Check sheet for the modelled part. Datum: model origin and axes. Units: mm. A direction names the side the tool comes from. Give positions to 0.01 mm unless a question says otherwise; leave off trailing zeros. Write each loop counter-clockwise with the first axis right and the second up, starting at its lowest first coordinate (ties: lowest second). Pieces come first, ordered by that corner, then holes. Notation, with made-up numbers: M 8.5,14 L 28.5,14 A25 ccw 28.5,35 Z; hole C 35,-21 d7. An arc over 180 degrees is marked long. Write item = value, one per line. Start each with the question number.
1) Scan lines: L1, parallel to Z at x = 293, y = 302; L2, parallel to Y at x = 222, z = 1.5; L3, parallel to X at y = 108.5, z = 1. Record each from-to range of solid material in increasing order.
2) Sectioned sample at A-A, the plane y = 333. Record the cut outline in (x, z), then the cut area to 3 significant figures.
3) Sectioned sample at B-B, the plane z = -5. Record the cut outline in (x, y), then the cut area to 3 significant figures.
4) Draft check along Y on faces 1 (the face through (281.901, 335.277, 1.479)), 2 (the face through (267.89, 313.772, 1.479)), 3 (the face through (189.3, 351.9, 1.5)), 4 (the face through (398.584, 56.784, 1.479)). Enter one of: pulls with the +Y half, pulls with the -Y half, needs draft (parallel to the pull), parting line crosses it, or undercut.
5) Set-up check for faces 5 (the face through (208.47, 362.55, 1.48)), 6 (the face through (346.985, 311.588, 1.479)), 7 (the face through (398.838, 182.595, -14.133)): record each of +Z, -Z, +X, -X, +Y, -Y from which the full face is reachable in a straight line by a thin tool's end or side.
6) Gauge pin test, flat ends, axial feed: pin 1 (5 mm diameter, centred on y = 116, z = -8.5, fed in from +X); pin 2 (3 mm diameter, centred on y = 113, z = -23, fed in from -X); pin 3 (6 mm diameter, centred on y = 322, z = -5.5, fed in from -X); pin 4 (4 mm diameter, centred on x = 312, y = 281, fed in from -Z). Record the tip position at first contact, or that the pin passes through.
from build123d import *

# Parameters (mm, degrees)
RESSALTO_EXTRUS_O1_DEPTH        = 3
ARESTA_FLANGE1_STRIP_W          = 13.8
ARESTA_FLANGE1_STRIP_H          = 3
ARESTA_FLANGE1_STRIP_CUT_DEPTH  = 248.223813341
ARESTA_FLANGE1_RELIEF_W         = 15.3
ARESTA_FLANGE1_RELIEF_H         = 1.5
ARESTA_FLANGE1_RELIEF_CUT_DEPTH = 3
ARESTA_FLANGE1_DEPTH            = 248.223813341


# Sheet-metal steps are written as plain solids
with BuildPart() as part:
    # Esboço29 → Ressalto-extrusão1 (new body)
    with BuildSketch(Plane.XY):
        with BuildLine():
            Line((423.645620755, 59.178719541), (380.542007914, 303.631455401))
            ThreePointArc((380.542007914, 303.631455401), (376.166741716, 313.014244041), (367.686255721, 318.952344263))
            Line((367.686255721, 318.952344263), (235.026475013, 367.236555725))
            ThreePointArc((235.026475013, 367.236555725), (228.186072146, 368.44270331), (221.34566928, 367.236555725))
            Line((221.34566928, 367.236555725), (195.221638123, 357.728185985))
            ThreePointArc((195.221638123, 357.728185985), (189.244913348, 351.75146121), (189.981585518, 343.331259777))
            Line((189.981585518, 343.331259777), (268.150737271, 207.938317356))
            ThreePointArc((268.150737271, 207.938317356), (270.383115212, 205.277872925), (273.390789876, 203.541391148))
            Line((273.390789876, 203.541391148), (294.669915314, 195.796422877))
            ThreePointArc((294.669915314, 195.796422877), (297.677589977, 194.059941101), (299.909967918, 191.399496669))
            Line((299.909967918, 191.399496669), (372.923716413, 64.935974625))
            ThreePointArc((372.923716413, 64.935974625), (375.848206088, 61.744454182), (379.847488675, 60.087897095))
            Line((379.847488675, 60.087897095), (417.853341101, 53.386439887))
            ThreePointArc((417.853341101, 53.386439887), (422.257115895, 54.774944746), (423.645620755, 59.178719541))
        make_face()
        with BuildLine():
            Line((243.325022214, 329.098265065), (239.916324262, 348.429951789))
            ThreePointArc((239.916324262, 348.429951789), (239.041271023, 350.306509517), (237.345173823, 351.494129561))
            Line((237.345173823, 351.494129561), (232.47795712, 353.265651565))
            ThreePointArc((232.47795712, 353.265651565), (231.109876546, 353.506881082), (229.741795973, 353.265651565))
            Line((229.741795973, 353.265651565), (204.889458572, 344.220140499))
            ThreePointArc((204.889458572, 344.220140499), (202.257539145, 340.461370016), (204.889458572, 336.702599533))
            Line((204.889458572, 336.702599533), (238.017710629, 324.644901871))
            ThreePointArc((238.017710629, 324.644901871), (241.956941641, 325.339494581), (243.325022214, 329.098265065))
        make_face(mode=Mode.SUBTRACT)
        with BuildLine():
            Line((249.39887944, 340.721872869), (252.807577392, 321.390186145))
            ThreePointArc((252.807577392, 321.390186145), (253.682630632, 319.513628417), (255.378727831, 318.326008373))
            Line((255.378727831, 318.326008373), (280.757120558, 309.089028826))
            ThreePointArc((280.757120558, 309.089028826), (282.125201132, 308.847799309), (283.493281705, 309.089028826))
            Line((283.493281705, 309.089028826), (308.345619106, 318.134539892))
            ThreePointArc((308.345619106, 318.134539892), (310.977538533, 321.893310376), (308.345619106, 325.652080859))
            Line((308.345619106, 325.652080859), (254.706191026, 345.175236063))
            ThreePointArc((254.706191026, 345.175236063), (250.766960014, 344.480643352), (249.39887944, 340.721872869))
        make_face(mode=Mode.SUBTRACT)
        with BuildLine():
            Line((328.999893161, 317.138658679), (304.14755576, 308.093147613))
            ThreePointArc((304.14755576, 308.093147613), (301.515636333, 304.33437713), (304.14755576, 300.575606647))
            Line((304.14755576, 300.575606647), (362.485446944, 279.342350725))
            ThreePointArc((362.485446944, 279.342350725), (366.424677956, 280.036943436), (367.79275853, 283.795713919))
            Line((367.79275853, 283.795713919), (364.384060578, 303.127400644))
            ThreePointArc((364.384060578, 303.127400644), (363.509007338, 305.003958372), (361.812910139, 306.191578416))
            Line((361.812910139, 306.191578416), (331.736054308, 317.138658679))
            ThreePointArc((331.736054308, 317.138658679), (330.367973734, 317.379888196), (328.999893161, 317.138658679))
        make_face(mode=Mode.SUBTRACT)
    extrude(amount=RESSALTO_EXTRUS_O1_DEPTH)

    # Aresta-Flange1 strip (across the edge) → Aresta-Flange1 strip cut (cut)
    with BuildSketch(Plane(origin=(380.542007914, 303.631455401, 0), x_dir=(-0.9848077530122086, -0.17364817766692797, -3.491481338843133e-15), z_dir=(0.17364817766692797, -0.9848077530122086, 0))):
        with Locations((-3, -1.5)):
            Rectangle(ARESTA_FLANGE1_STRIP_W, ARESTA_FLANGE1_STRIP_H)
    extrude(amount=ARESTA_FLANGE1_STRIP_CUT_DEPTH, mode=Mode.SUBTRACT)

    # Aresta-Flange1 relief (on the sheet) → Aresta-Flange1 relief cut (cut)
    with BuildSketch(Plane(origin=(376.701257678, 302.954227508, 0), x_dir=(-0.9848077530122086, -0.17364817766692797, -6.982962677686267e-15), z_dir=(0, 0, -1))):
        with Locations((-6.15, 0.75)):
            Rectangle(ARESTA_FLANGE1_RELIEF_W, ARESTA_FLANGE1_RELIEF_H)
        with Locations((-6.15, -248.973813341)):
            Rectangle(ARESTA_FLANGE1_RELIEF_W, ARESTA_FLANGE1_RELIEF_H)
    extrude(amount=-ARESTA_FLANGE1_RELIEF_CUT_DEPTH, mode=Mode.SUBTRACT)

    # Aresta-Flange1 section (across the edge) → Aresta-Flange1 (add)
    with BuildSketch(Plane(origin=(380.542007914, 303.631455401, 0), x_dir=(-0.9848077530122086, -0.17364817766692797, -3.491481338843133e-15), z_dir=(0.17364817766692797, -0.9848077530122086, 0))):
        with BuildLine():
            Line((0, 0.9), (0, 27))
            Line((0, 27), (3, 27))
            Line((3, 27), (3, 0.9))
            ThreePointArc((3, 0.9), (3.263603897, 0.263603897), (3.9, 0))
            Line((3.9, 0), (3.9, -3))
            ThreePointArc((3.9, -3), (1.142283553, -1.857716447), (0, 0.9))
        make_face()
    extrude(amount=ARESTA_FLANGE1_DEPTH)


solid = part.part
Data:
q1.L1 = 0 to 3
q1.L2 = 287.87 to 330.47, 350.45 to 367.46
q1.L3 = 347.77 to 414.45
q2.outline = M 195.95,0 L 215.06,0 L 215.06,3 L 195.95,3 Z; M 242.64,0 L 250.76,0 L 250.76,3 L 242.64,3 Z; M 288.16,0 L 329.09,0 L 329.09,3 L 288.16,3 Z
q2.area = 205 mm2
q3.outline = M 377.59,303.11 L 420.69,58.66 L 423.65,59.18 L 380.54,303.63 Z
q3.area = 745 mm2
q4.face_1 = undercut
q4.face_2 = undercut
q4.face_3 = parting line crosses it
q4.face_4 = pulls with the -Y half
q5.face_5 = +Z, -Z, -X, +Y
q5.face_6 = +Z, -Z
q5.face_7 = -Z, -X, -Y
q6.pin_1 = 414.07
q6.pin_2 = 410.84
q6.pin_3 = through
q6.pin_4 = 0
